Verification items for the finished model (mm, model axes). A direction names the side the tool comes from. Round coordinates to 2 decimals unless told otherwise and drop trailing zeros. Loops run counter-clockwise (first coordinate to the right, second up) from the corner with the lowest first, then second, coordinate; pieces in that order, holes last. Notation, with made-up numbers: M 56.25,67.5 L 105.25,67.5 A31 ccw 105.25,94.5 Z; hole C 51,-10.75 d2. An arc over 180 degrees is marked long. One line per item, written item: value.
from build123d import *

# Parameters (mm, degrees)
F0_W      = 101.6
F0_H      = 101.6
F1_DEPTH  = 101.6
F2_R      = 12.7
F3_DEPTH  = 2.54
F4_R      = 12.7
F5_DEPTH  = 2.54
F6_R      = 12.7
F7_DEPTH  = 2.54
F8_R      = 12.7
F9_DEPTH  = 2.54
F10_R     = 12.7
F11_DEPTH = 2.54
F12_R     = 12.7
F13_DEPTH = 2.54


with BuildPart() as f1:
    # F0 (on Top) → F1 (new body)
    with BuildSketch(Plane.XY):
        with Locations((-4.690753, -12.038526)):
            Rectangle(F0_W, F0_H)
    extrude(amount=F1_DEPTH)

    # F2 (on face) → F3 (cut)
    with BuildSketch(Plane.XZ.offset(62.838526)):
        with Locations((-37.710753, 17.78)):
            Circle(F2_R)
        with Locations((-37.710753, 50.8)):
            Circle(F2_R)
        with Locations((-37.710753, 83.82)):
            Circle(F2_R)
        with Locations((28.329247, 17.78)):
            Circle(F2_R)
        with Locations((28.329247, 50.8)):
            Circle(F2_R)
        with Locations((28.329247, 83.82)):
            Circle(F2_R)
    extrude(amount=-F3_DEPTH, mode=Mode.SUBTRACT)

    # F4 (on face) → F5 (cut)
    with BuildSketch(Plane(origin=(0, 38.761474, 0), x_dir=(-1, 0, 0), z_dir=(0, 1, 0))):
        with Locations((4.690753, 50.8)):
            Circle(F4_R)
    extrude(amount=-F5_DEPTH, mode=Mode.SUBTRACT)

    # F6 (on face) → F7 (cut)
    with BuildSketch(Plane(origin=(-55.490753, 0, 0), x_dir=(0, -1, 0), z_dir=(-1, 0, 0))):
        with Locations((-20.981474, 83.82)):
            Circle(F6_R)
        with Locations((12.038526, 50.8)):
            Circle(F6_R)
        with Locations((-20.981474, 17.78)):
            Circle(F6_R)
        with Locations((45.058526, 83.82)):
            Circle(F6_R)
        with Locations((45.058526, 17.78)):
            Circle(F6_R)
    extrude(amount=-F7_DEPTH, mode=Mode.SUBTRACT)

    # F8 (on face) → F9 (cut)
    with BuildSketch(Plane.YZ.offset(46.109247)):
        with Locations((-45.058526, 83.82)):
            Circle(F8_R)
        with Locations((20.981474, 17.78)):
            Circle(F8_R)
    extrude(amount=-F9_DEPTH, mode=Mode.SUBTRACT)

    # F10 (on face) → F11 (cut)
    with BuildSketch(Plane.XY.offset(101.6)):
        with Locations((-37.710753, 20.981474)):
            Circle(F10_R)
        with Locations((-4.690753, -12.038526)):
            Circle(F10_R)
        with Locations((28.329247, -45.058526)):
            Circle(F10_R)
    extrude(amount=-F11_DEPTH, mode=Mode.SUBTRACT)

    # F12 (on face) → F13 (cut)
    with BuildSketch(Plane(origin=(0, 0, 0), x_dir=(1, 0, 0), z_dir=(0, 0, -1))):
        with Locations((-37.710753, 45.058526)):
            Circle(F12_R)
        with Locations((-37.710753, -20.981474)):
            Circle(F12_R)
        with Locations((28.329247, 45.058526)):
            Circle(F12_R)
        with Locations((28.329247, -20.981474)):
            Circle(F12_R)
    extrude(amount=-F13_DEPTH, mode=Mode.SUBTRACT)


solid = f1.part
(1) Sectioned sample at D-D on z = 50.8. Enter the section's corners in (x, y), and give its area (3 significant figures).
Completed:
outline: M -55.49,-62.84 L -50.41,-62.84 L -50.41,-60.3 L -25.01,-60.3 L -25.01,-62.84 L 15.63,-62.84 L 15.63,-60.3 L 41.03,-60.3 L 41.03,-62.84 L 46.11,-62.84 L 46.11,38.76 L 8.01,38.76 L 8.01,36.22 L -17.39,36.22 L -17.39,38.76 L -55.49,38.76 L -55.49,0.66 L -52.95,0.66 L -52.95,-24.74 L -55.49,-24.74 Z
area: 10,100 mm^2
(2) Depth check by flat-ended pin: pin 1 Ø12.5 at (y, z) = (26.5, 17.5) entering from +X; pin 2 Ø2 at (y, z) = (-43.5, 77.5) entering from -X; pin 3 Ø2 at (x, y) = (-41.5, 27.5) entering from -Z. Enter the tip coordinate at first touch or a pass-through.
Completed:
pin 1: stops at x = 43.57
pin 2: stops at x = -52.95
pin 3: stops at z = 2.54
(3) Thickness scan on L1, parallel to Y at x = -30, z = 93.5; L2, parallel to Y at x = -11.5, z = 58; L3, parallel to Z at x = -35, y = 13. Record the ranges inside material, lowest first. Write a range as from..to.
Completed:
L1: y = -60.3..38.76
L2: y = -62.84..36.22
L3: z = 2.54..99.06
(4) Mould release check, pull along Y, two halves, no side actions. Record for faces 4 (the face through (-31.85, 9.714, 100.348)), 5 (the face through (40.443, -61.586, 87.635)), 6 (the face through (28, -60.299, 51)): +Y half, -Y half, draft (parallel to the pull), parting line (faces both ways), or undercut.
Completed:
face 4: undercut
face 5: draft
face 6: -Y half
(5) Sectioned sample at A-A on z = 17.78. Enter the section's corners in (x, y), and give its area (4 significant figures).
Completed:
outline: M -55.49,-62.84 L -50.41,-62.84 L -50.41,-60.3 L -25.01,-60.3 L -25.01,-62.84 L 15.63,-62.84 L 15.63,-60.3 L 41.03,-60.3 L 41.03,-62.84 L 46.11,-62.84 L 46.11,8.28 L 43.57,8.28 L 43.57,33.68 L 46.11,33.68 L 46.11,38.76 L -55.49,38.76 L -55.49,33.68 L -52.95,33.68 L -52.95,8.28 L -55.49,8.28 L -55.49,-32.36 L -52.95,-32.36 L -52.95,-57.76 L -55.49,-57.76 Z
area: 10,000 mm^2
(6) Tool access check on faces 1 (the face through (-54.24, -34.98, 10.05)), 2 (the face through (44.86, -54.42, 92.4)), 3 (the face through (28, 21, 2.54)). Record the directions out of +Z, -Z, +X, -X, +Y, -Y that give a thin tool (end or side, any length) a straight path to the whole face; none if there is none.
Completed:
face 1: -X
face 2: +X
face 3: -Z
(7) Sectioned sample at B-B on y = 14. Enter the section's corners in (x, z), and give its area (4 significant figures).
Completed:
outline: M -55.49,0 L -48.32,0 L -48.32,2.54 L -27.1,2.54 L -27.1,0 L 17.72,0 L 17.72,2.54 L 38.94,2.54 L 38.94,0 L 46.11,0 L 46.11,7.17 L 43.57,7.17 L 43.57,28.39 L 46.11,28.39 L 46.11,101.6 L -27.1,101.6 L -27.1,99.06 L -48.32,99.06 L -48.32,101.6 L -55.49,101.6 L -55.49,94.43 L -52.95,94.43 L -52.95,73.21 L -55.49,73.21 L -55.49,28.39 L -52.95,28.39 L -52.95,7.17 L -55.49,7.17 Z
area: 10,000 mm^2
(8) Sectioned sample at C-C on x = 35.5. Enter the section's corners in (y, z).
Completed:
outline: M -62.84,0 L -55.54,0 L -55.54,2.54 L -34.58,2.54 L -34.58,0 L 10.5,0 L 10.5,2.54 L 31.46,2.54 L 31.46,0 L 38.76,0 L 38.76,101.6 L -34.58,101.6 L -34.58,99.06 L -55.54,99.06 L -55.54,101.6 L -62.84,101.6 L -62.84,94.3 L -60.3,94.3 L -60.3,73.34 L -62.84,73.34 L -62.84,61.28 L -60.3,61.28 L -60.3,40.32 L -62.84,40.32 L -62.84,28.26 L -60.3,28.26 L -60.3,7.3 L -62.84,7.3 Z
